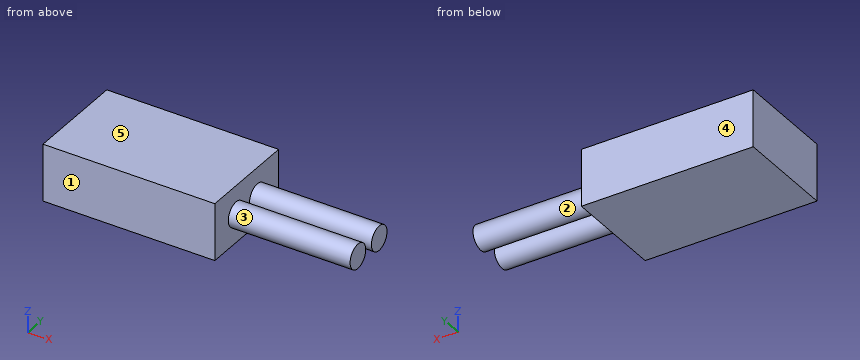
from build123d import *

# Parameters (mm, degrees)
SKETCH1_W           = 70.1
SKETCH1_H           = 40.8
BOSS_EXTRUDE1_DEPTH = 23.3
SKETCH2_R           = 5
BOSS_EXTRUDE2_DEPTH = 49.7


with BuildPart() as part:
    # Sketch1 → Boss-Extrude1 (new body)
    with BuildSketch(Plane.XY):
        with Locations((35.05, 20.4)):
            Rectangle(SKETCH1_W, SKETCH1_H)
    extrude(amount=BOSS_EXTRUDE1_DEPTH)

    # Sketch2 → Boss-Extrude2 (add)
    with BuildSketch(Plane(origin=(70.1, 0, 0), x_dir=(0, 0, -1), z_dir=(1, 0, 0))):
        with Locations((-11.65, 27.2)):
            Circle(SKETCH2_R)
        with Locations(Location((-11.65, 13.6, 0), (0, 0, 180))):
            Circle(SKETCH2_R)
    extrude(amount=BOSS_EXTRUDE2_DEPTH)


solid = part.part
Build history of the part. All positions in model axes, mm. Face numbers are marked on the shaded views. A direction names the side the tool comes from. Coordinates: 2 decimals unless noted, no trailing zeros. Order: outer loops, then holes, each group sorted by start corner. A loop starts at its lowest first (then second) coordinate and runs counter-clockwise, first axis right, second up. Notation, with made-up numbers: (61, 47) -> (65, 47) arc R26 ccw to (65, 69) -> close; hole circle Ø10 at (22.25, 24). An arc over 180 degrees is marked (long way). One line per item, written item: value.
(1) Tool access for the marked faces 1 and 2: list every direction of +Z, -Z, +X, -X, +Y, -Y with a clear straight run to the whole face (end or side of a thin tool).
Checked values:
face 1: +Z, -Z, +X, -X, -Y
face 2: +X
(2) Drop a flat-ended pin along its axis: pin 1 Ø4 at (x, y) = (58.5, 35) entering from -Z. Give the stop position or say it passes through.
Checked values:
pin 1: z = 0
(3) Mould opens along Y. For the marked faces 3, 4 and 5 say: pulls with the +Y half, pulls with the -Y half, needs draft (parallel to the pull), parting line crosses it, or undercut.
Checked values:
face 3: undercut
face 4: pulls with the +Y half
face 5: needs draft
(4) Slice it at B-B, the plane y = 27.2. List the corners of the cut face in (x, z), plus the area to 3 significant figures.
Checked values:
outline: (0, 0) -> (70.1, 0) -> (70.1, 6.65) -> (119.8, 6.65) -> (119.8, 16.65) -> (70.1, 16.65) -> (70.1, 23.3) -> (0, 23.3) -> close
area: 2,130 mm2
(5) Slice it at D-D, the plane y = 10. List the corners of the cut face in (x, z).
Checked values:
outline: (0, 0) -> (70.1, 0) -> (70.1, 8.18) -> (119.8, 8.18) -> (119.8, 15.12) -> (70.1, 15.12) -> (70.1, 23.3) -> (0, 23.3) -> close
(6) Slice it at C-C, the plane x = 78. List the corners of the cut face in (y, z), plus the area to 3 significant figures.
Checked values:
outline: circle Ø10 at (13.6, 11.65); circle Ø10 at (27.2, 11.65)
area: 157 mm2
(7) Slice it at A-A, the plane z = 14.25. List the corners of the cut face in (x, y).
Checked values:
outline: (0, 0) -> (70.1, 0) -> (70.1, 9.33) -> (119.8, 9.33) -> (119.8, 17.87) -> (70.1, 17.87) -> (70.1, 22.93) -> (119.8, 22.93) -> (119.8, 31.47) -> (70.1, 31.47) -> (70.1, 40.8) -> (0, 40.8) -> close
(8) Probe line 1 (X direction, y = 18, z = 17.75); line 2 (Y direction, x = 115, z = 11.75); line 3 (Y direction, x = 111.5, z = 8). List the from-to ranges inside material, lowest first. Write a range as [from, to].
Checked values:
line 1: [0, 70.1]
line 2: [8.6, 18.6], [22.2, 32.2]
line 3: [10.18, 17.02], [23.78, 30.62]
